Build history of the part. All positions in model axes, mm. Give positions to 0.01 mm unless a question says otherwise; leave off trailing zeros. Order: outer loops, then holes, each group sorted by start corner. A loop starts at its lowest first (then second) coordinate and runs counter-clockwise, first axis right, second up. Notation, with made-up numbers: M 5,8 L 31,8 A31 ccw 31,42 Z; hole C 38,-2.5 d5. An arc over 180 degrees is marked long. Answer as CSV lines item,"result".
Autodesk Inventor part; units mm, degrees
ref_plane "YZ Plane" through (0, 0, 0) normal (1, 0, 0) x (0, 1, 0)
ref_plane "XZ Plane" through (0, 0, 0) normal (0, 1, 0) x (-1, 0, 0)
ref_plane "XY Plane" through (0, 0, 0) normal (0, 0, 1) x (1, 0, 0)
sketch "Sketch1" plane through (0, 0, 0) normal (0, 0, 1) x (1, 0, 0)
  line L0 (-158.5, 220) -> (158.5, 220)
  line L1 (158.5, 220) -> (158.5, -220)
  line L2 (158.5, -220) -> (-158.5, -220)
  line L3 (-158.5, -220) -> (-158.5, 220)
  line L4 (-153.5, 215) -> (153.5, 215) construction
  line L5 (153.5, 215) -> (153.5, -215) construction
  line L6 (153.5, -215) -> (-153.5, -215) construction
  line L7 (-153.5, -215) -> (-153.5, 215) construction
  circle A0 centre (-153.5, 215) radius 2
  circle A1 centre (153.5, 215) radius 2
  circle A2 centre (153.5, -215) radius 2
  circle A3 centre (-153.5, -215) radius 2
  point P0 (0, 0)
  point P1 (0, 220)
  point P2 (-158.5, 0)
  point P3 (0, 215)
  point P4 (-153.5, 0)
  dimension "d0" = 440
  dimension "d1" = 317
  dimension "d3" = 5
  dimension "d4" = 5
  dimension "d5" = 4
extrude "Extrusion1" add sketch "Sketch1" along normal blind 4
sketch "Sketch3" plane through (0, 0, 0) normal (0, 0, -1) x (-1, 0, 0)
  line L0 (90, -220) -> (-90, -220)
  line L1 (-90, -220) -> (-90, 220)
  line L2 (-90, 220) -> (90, 220)
  line L3 (90, 220) -> (90, -220)
  line L4 (158.5, -220) -> (-158.5, -220)
  line L5 (-158.5, 220) -> (158.5, 220)
  line L6 (90, -40) -> (-90, -40)
  line L7 (-90, -40) -> (-90, 40)
  line L8 (-90, 40) -> (90, 40)
  line L9 (90, 40) -> (90, -40)
  point P0 (0, 0)
  point P1 (0, -220)
  point P2 (-90, 0)
  dimension "d11" = 180
  dimension "d12" = 80
extrude "Extrusion3" cut sketch "Sketch3" against normal through all contours L0 L1 L6 L3 | L8 L1 L2 L3
sketch "Sketch5" plane through (0, 0, 4) normal (0, 0, 1) x (1, 0, 0)
  line L0 (158.5, -240) -> (90, -240)
  line L1 (90, -240) -> (90, -220)
  line L2 (90, -220) -> (158.5, -220)
  line L3 (158.5, -220) -> (158.5, -240)
  line L4 (158.5, 220) -> (90, 220)
  line L5 (158.5, -220) -> (158.5, 220)
  line L6 (90, 220) -> (90, 40)
  circle A0 centre (153.5, -230) radius 2.5
  circle A1 centre (103.5, -230) radius 2.5
  line L7 (90, -220) -> (158.5, -220)
  point P0 (0, 0)
  point P1 (124.25, 201.6144)
  point P2 (124.25, -240)
  point P3 (90, -230)
  dimension "d21" = 20
  dimension "d22" = 5
  dimension "d24" = 50
  dimension "d34" = 5
extrude "Extrusion5" add sketch "Sketch5" against normal up to surface (4 mm away)
sketch "Sketch6" plane through (0, 0, 0) normal (0, 0, -1) x (-1, 0, 0)
  circle A0 centre (119.5, -78) radius 2.1
  circle A1 centre (147.5, -78) radius 2.1
  circle A2 centre (119.5, -57) radius 2.1
  circle A3 centre (147.5, -57) radius 2.1
  line L0 (152.5, -85) -> (142.5, -85)
  line L1 (142.5, -85) -> (142.5, -50)
  line L2 (142.5, -50) -> (152.5, -50)
  line L3 (152.5, -50) -> (152.5, -85)
  line L4 (137.5, -85) -> (129.5, -85)
  line L5 (129.5, -85) -> (129.5, -50)
  line L6 (129.5, -50) -> (137.5, -50)
  line L7 (137.5, -50) -> (137.5, -85)
  line L8 (124.5, -85) -> (114.5, -85)
  line L9 (114.5, -85) -> (114.5, -50)
  line L10 (114.5, -50) -> (124.5, -50)
  line L11 (124.5, -50) -> (124.5, -85)
  circle A4 centre (119.5, 57) radius 2.1
  circle A5 centre (147.5, 57) radius 2.1
  circle A6 centre (119.5, 78) radius 2.1
  circle A7 centre (147.5, 78) radius 2.1
  line L12 (152.5, 50) -> (142.5, 50)
  line L13 (142.5, 50) -> (142.5, 85)
  line L14 (142.5, 85) -> (152.5, 85)
  line L15 (152.5, 85) -> (152.5, 50)
  line L16 (137.5, 50) -> (129.5, 50)
  line L17 (129.5, 50) -> (129.5, 85)
  line L18 (129.5, 85) -> (137.5, 85)
  line L19 (137.5, 85) -> (137.5, 50)
  line L20 (124.5, 50) -> (114.5, 50)
  line L21 (114.5, 50) -> (114.5, 85)
  line L22 (114.5, 85) -> (124.5, 85)
  line L23 (124.5, 85) -> (124.5, 50)
  circle A8 centre (1, 0) radius 2.5
  circle A9 centre (30, 0) radius 2.5
  line L24 (10.5, -12) -> (30.5, -12)
  line L25 (30.5, -12) -> (30.5, -5)
  line L26 (30.5, -5) -> (10.5, -5)
  line L27 (10.5, -5) -> (10.5, -12)
  line L28 (-50, -15.5) -> (40, -15.5)
  line L29 (40, 15.5) -> (40, -15.5)
  line L30 (40, 15.5) -> (-50, 15.5)
  line L31 (-50, -15.5) -> (-50, 15.5)
  line L32 (30.5, 12) -> (10.5, 12)
  line L33 (10.5, 12) -> (10.5, 5)
  line L34 (10.5, 5) -> (30.5, 5)
  line L35 (30.5, 5) -> (30.5, 12)
  circle A10 centre (-16, -10.5) radius 3
  circle A11 centre (-44, -10.5) radius 3
  circle A12 centre (-44, 10.5) radius 3
  circle A13 centre (-16, 10.5) radius 3
  circle A14 centre (-119.5, -57) radius 2.1
  circle A15 centre (-147.5, -57) radius 2.1
  circle A16 centre (-119.5, -78) radius 2.1
  circle A17 centre (-147.5, -78) radius 2.1
  line L36 (-152.5, -50) -> (-142.5, -50)
  line L37 (-142.5, -50) -> (-142.5, -85)
  line L38 (-142.5, -85) -> (-152.5, -85)
  line L39 (-152.5, -85) -> (-152.5, -50)
  line L40 (-137.5, -50) -> (-129.5, -50)
  line L41 (-129.5, -50) -> (-129.5, -85)
  line L42 (-129.5, -85) -> (-137.5, -85)
  line L43 (-137.5, -85) -> (-137.5, -50)
  line L44 (-124.5, -50) -> (-114.5, -50)
  line L45 (-114.5, -50) -> (-114.5, -85)
  line L46 (-114.5, -85) -> (-124.5, -85)
  line L47 (-124.5, -85) -> (-124.5, -50)
  circle A18 centre (-147.5, 57) radius 2.1
  circle A19 centre (-119.5, 57) radius 2.1
  circle A20 centre (-147.5, 78) radius 2.1
  circle A21 centre (-119.5, 78) radius 2.1
  line L48 (-114.5, 50) -> (-124.5, 50)
  line L49 (-124.5, 50) -> (-124.5, 85)
  line L50 (-124.5, 85) -> (-114.5, 85)
  line L51 (-114.5, 85) -> (-114.5, 50)
  line L52 (-129.5, 50) -> (-137.5, 50)
  line L53 (-137.5, 50) -> (-137.5, 85)
  line L54 (-137.5, 85) -> (-129.5, 85)
  line L55 (-129.5, 85) -> (-129.5, 50)
  line L56 (-142.5, 50) -> (-152.5, 50)
  line L57 (-152.5, 50) -> (-152.5, 85)
  line L58 (-152.5, 85) -> (-142.5, 85)
  line L59 (-142.5, 85) -> (-142.5, 50)
  point P0 (0, 0)
hole "Hole1" at (-147.5, -78, 0) at (-119.5, -78, 0) at (-119.5, -57, 0) at (-147.5, -57, 0) at (-30, 0, 0) at (0, 0, 0) at (16, -10.5, 0) at (44, -10.5, 0) at (44, 10.5, 0) at (16, 10.5, 0) at (-119.5, 57, 0) at (-119.5, 78, 0) at (-147.5, 78, 0) at (-147.5, 57, 0) at (119.5, 57, 0) at (147.5, 57, 0) at (147.5, 78, 0) at (119.5, 78, 0) at (147.5, -78, 0) at (119.5, -78, 0) at (119.5, -57, 0) at (147.5, -57, 0) direction (0, 0, 1) diameter 5 end through all
sketch "Sketch7" plane through (0, 0, 0) normal (0, 0, -1) x (-1, 0, 0)
  line L0 (-60, -15.1293) -> (-60, -45.1293)
  line L1 (-71, -45.1293) -> (-60, -45.1293)
  line L2 (-71, -45.1293) -> (-71, -15.1293)
  line L3 (-71, -15.1293) -> (-60, -15.1293)
  circle A0 centre (88, -28) radius 2
  circle A1 centre (88, -20) radius 2
  line L4 (-90, -40) -> (90, -40)
  circle A2 centre (88, -5) radius 7.5
  circle A3 centre (76, -10) radius 3
  circle A4 centre (103, -10) radius 3
  line L5 (84.5, -12.7391) -> (91.5, -12.7391)
  line L6 (84.5, -12.7391) -> (84.5, -22.7391)
  line L7 (93.5, -12.7391) -> (93.5, -22.7391)
  line L8 (-107, -6) -> (107, -6)
  line L9 (-107, -220) -> (-107, -6)
  line L10 (107, -220) -> (-107, -220)
  line L11 (107, -6) -> (107, -220)
  circle A5 centre (104.5, -217.5) radius 1.5
  circle A6 centre (-104.5, -217.5) radius 1.5
  circle A7 centre (-104.5, -8.5) radius 1.5
  circle A8 centre (104.5, -8.5) radius 1.5
  point P0 (0, 0)
  dimension "d35" = 4
  dimension "d37" = 8
  dimension "d38" = 12
  dimension "d39" = 15
  dimension "d40" = 35
  dimension "d41" = 6
  dimension "d42" = 12
  dimension "d43" = 15
  dimension "d44" = 5
  dimension "d47" = 5.5
extrude "Extrusion6" cut sketch "Sketch7" against normal through all contours A0 | A1 | A2 L8 | L8 A2 | A3 | A4 A8 | A8 A4 picked at (101.8731, -11.3773) picked at (104.2239, -7.9666)
equation "\"d43\" = d39"
properties part number "0008-10-018 Suport Heated Bed" material "Aluminum 6061"
Item 1: Pull direction Y, two halves, no side cores. Call faces 1 (the flat face through (-2, -7, 4)), 2 (the cylindrical face through (-80.507, -4.67, 1.972)): released by +Y, released by -Y, zero draft, split by the parting line, or undercut.
Geometry says:
face 1,"zero draft"
face 2,"undercut"
Item 2: Band-saw the part on A-A (y = -127). Give the cut face in (x, z).
Geometry says:
outline,"M -158.5,0 L -90,0 L -90,4 L -158.5,4 Z; M 90,0 L 158.5,0 L 158.5,4 L 90,4 Z"
Item 3: Band-saw the part on B-B (z = 1.25). State how many separate pieces and enclosed holes the cut face has, and give its area (3 significant figures).
Geometry says:
separate pieces,"1"
enclosed holes,"33"
area,"75,300 mm2"
Item 4: Band-saw the part on C-C (x = 59.5). Give the cut face in (y, z).
Geometry says:
outline,"M -40,0 L 40,0 L 40,4 L -40,4 Z"
Item 5: Drop flat-ended pins along their axis: pin 1 (2 mm diameter, centred on x = -43.5, z = 1.5, fed in from -Y); pin 2 (1.2 mm diameter, centred on x = 34, z = 2.5, fed in from +Y). Give the stop position or say it passes through.
Geometry says:
pin 1,"stops at y = -40"
pin 2,"stops at y = 40"
Item 6: Probe line 1 along X through (y, z) = (78, 3.1); line 2 along Y through (x, z) = (147.5, 2.7); line 3 along Y through (x, z) = (-119.5, 2.2). List the from-to ranges inside material, lowest first. Write a range as from..to.
Geometry says:
line 1,"x = -158.5..-150, -145..-122, -117..-90, 90..117, 122..145, 150..158.5"
line 2,"y = -240..-80.5, -75.5..-59.5, -54.5..54.5, 59.5..75.5, 80.5..220"
line 3,"y = -220..-80.5, -75.5..-59.5, -54.5..54.5, 59.5..75.5, 80.5..220"
